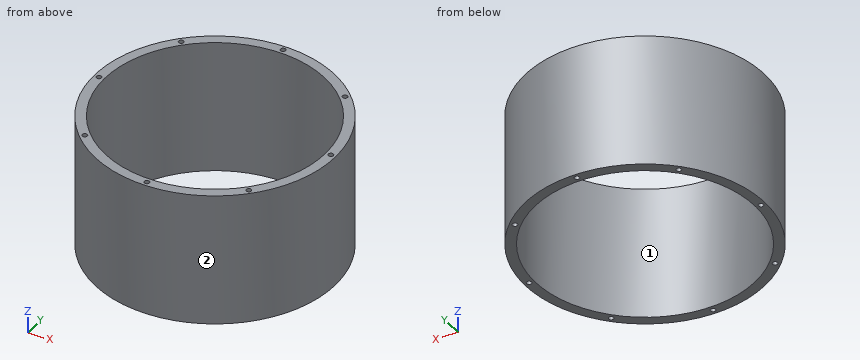
from build123d import *

# Parameters (mm, degrees)
F0_R     = 36
F1_DEPTH = 40
F2_R     = 33
F3_DEPTH = 40.001
F5_D     = 1.5


with BuildPart() as f1:
    # F0 (on Top) → F1 (new body)
    with BuildSketch(Plane.XY):
        Circle(F0_R)
    extrude(amount=F1_DEPTH)

    # F2 (on Top) → F3 (cut, through all)
    with BuildSketch(Plane.XY):
        Circle(F2_R)
    extrude(amount=F3_DEPTH, mode=Mode.SUBTRACT)

    # F5 (through all)
    with Locations(Plane(origin=(0, 0, 0), x_dir=(1, 0, 0), z_dir=(0, 0, -1))):
        with Locations((0, 34.5), (-24.3951839509, 24.3951839509), (-34.5, 0), (24.3951839509, 24.3951839509), (-24.3951839509, -24.3951839509), (0, -34.5), (24.3951839509, -24.3951839509), (34.5, 0)):
            Hole(F5_D / 2)


solid = f1.part
Could you check a few things on this model? Use its own coordinates, in mm. Face numbers are marked on the shaded views. Give positions to 0.01 mm unless a question says otherwise; leave off trailing zeros. Loops run counter-clockwise (first coordinate to the right, second up) from the corner with the lowest first, then second, coordinate; pieces in that order, holes last. Notation, with made-up numbers: (-35.5, 50.5) -> (-31.5, 50.5) arc R15 cw to (-31.5, 79.5) -> close; hole circle Ø3 at (28, 69.25). An arc over 180 degrees is marked (long way). Answer as CSV lines item,"result". Start each with the question number.
(1) I'm going to push flat-ended pins straight in: pin 1 Ø12 at (y, z) = (-10.5, 23.5) entering from +X; pin 2 Ø12 at (x, z) = (-17.5, 19.5) entering from -Y; pin 3 Ø12 at (x, z) = (-8, 27) entering from +Y. Where does each tip first touch, or does it pass through?
(2) If we section it at A-A on y = -13: Write out the boundary of the cut face in (x, z).
(3) We'd pull the mould along Y, two halves only. Please class the marked faces 1 and 2: released by +Y, released by -Y, zero draft, split by the parting line, or undercut.
(4) If we section it at C-C on x = -10: Write out the boundary of the cut face in (y, z), then the cut area to 3 significant figures.
(5) I need wall thicknesses on probe 1 along Y at (x, z) = (0, 13); probe 2 along X at (y, z) = (24.5, 35); probe 3 along X at (y, z) = (13.5, 37.5). Which ranges of each line are inside material? Lowest first, please.
(6) If we section it at B-B on z = 5.5: Count the separate pieces of the cut face and the enclosed holes in it, then the cut area to 3 significant figures.
Computed:
1,pin 1,"stops at x = 35.72"
1,pin 2,"stops at y = -34.11"
1,pin 3,"stops at y = 35.94"
2,outline,"(-33.57, 0) -> (-30.33, 0) -> (-30.33, 40) -> (-33.57, 40) -> close; (30.33, 0) -> (33.57, 0) -> (33.57, 40) -> (30.33, 40) -> close"
3,face 1,"undercut"
3,face 2,"split by the parting line"
4,outline,"(-34.58, 0) -> (-31.45, 0) -> (-31.45, 40) -> (-34.58, 40) -> close; (31.45, 0) -> (34.58, 0) -> (34.58, 40) -> (31.45, 40) -> close"
4,area,"251 mm2"
5,probe 1,"y = -36 to -35.25, -33.75 to -33, 33 to 33.75, 35.25 to 36"
5,probe 2,"x = -26.38 to -25.14, -23.65 to -22.11, 22.11 to 23.65, 25.14 to 26.38"
5,probe 3,"x = -33.37 to -30.11, 30.11 to 33.37"
6,separate pieces,"1"
6,enclosed holes,"9"
6,area,"636 mm2"
